Check sheet for the modelled part. Datum: model origin and axes. Units: mm. A direction names the side the tool comes from. Round coordinates to 2 decimals unless told otherwise and drop trailing zeros. Order: outer loops, then holes, each group sorted by start corner. A loop starts at its lowest first (then second) coordinate and runs counter-clockwise, first axis right, second up.
Q1. Cross-section at C-C on x = -22. Record the cut outline in (y, z), then the cut area to 3 significant figures.
Q2. Cross-section at B-B on z = 2.5. Record the cut outline in (x, y), then the cut area to 3 significant figures.
Q3. Cross-section at A-A on y = 20.5. Record the cut outline in (x, z), then the cut area to 3 significant figures.
Q4. Depth check by flat-ended pin: P1, Ø2.5, axis at x = 4, z = 2.5, coming from the +Y side. Enter the tip coordinate at first touch or a pass-through.
Q5. Mould release check, pull along X, two halves, no side actions. Record for faces 1 (the flat face through (0, 14, 0)), 2 (the flat face through (0, 15.955, 4)), 3 (the flat face through (-29.21, 20, 4)): +X half, -X half, draft (parallel to the pull), parting line (faces both ways), or undercut.
Q6. Cross-section at D-D on x = -10.5. Record the cut outline in (y, z), then the cut area to 3 significant figures.
Q7. Scan lines: probe 1 along X at (y, z) = (20.5, 5); probe 2 along Y at (x, z) = (-5, 5); probe 3 along Y at (x, z) = (22, 5). Record each from-to range of solid material in increasing order.
Q8. Set-up check for faces 4 (the flat face through (16.51, 33, 4)), 5 (the flat face through (29.21, 19, 4)): record each of +Z, -Z, +X, -X, +Y, -Y from which the full face is reachable in a straight line by a thin tool's end or side.
from build123d import *

# Parameters (mm, degrees)
F1_DEPTH = 7.62


with BuildPart() as f1:
    # F0 (on Top) → F1 (new body)
    with BuildSketch(Plane.XY):
        with BuildLine():
            Line((-29.210002, 48.974563), (-29.210002, 15.954563))
            Line((-29.210002, 15.954563), (-22.860002, 15.954563))
            Line((-22.860002, 15.954563), (-22.860002, 29.926767))
            ThreePointArc((-22.860002, 29.926767), (-25.397797, 32.464563), (-22.860002, 35.002358))
            Line((-22.860002, 35.002358), (-22.860002, 48.974563))
            Line((-22.860002, 48.974563), (-29.210002, 48.974563))
        make_face()
        Polygon((-22.860002, 15.954563), (-29.210002, 15.954563), (-29.210002, -9.445437), (29.209998, -9.445437), (29.209998, 15.954563), (22.859998, 15.954563), (16.509998, 15.954563), (-16.510002, 15.954563), align=None)
        with BuildLine():
            Line((-22.860002, 29.926767), (-22.860002, 15.954563))
            Line((-22.860002, 15.954563), (-16.510002, 15.954563))
            Line((-16.510002, 15.954563), (-16.510002, 48.974563))
            Line((-16.510002, 48.974563), (-22.860002, 48.974563))
            Line((-22.860002, 48.974563), (-22.860002, 35.002358))
            ThreePointArc((-22.860002, 35.002358), (-21.065509, 34.259055), (-20.322206, 32.464563))
            ThreePointArc((-20.322206, 32.464563), (-21.065509, 30.67007), (-22.860002, 29.926767))
        make_face()
        with BuildLine():
            Line((16.509998, 48.974563), (16.509998, 15.954563))
            Line((16.509998, 15.954563), (22.859998, 15.954563))
            Line((22.859998, 15.954563), (22.859998, 29.928652))
            ThreePointArc((22.859998, 29.928652), (20.324087, 32.464563), (22.859998, 35.000474))
            Line((22.859998, 35.000474), (22.859998, 48.974563))
            Line((22.859998, 48.974563), (16.509998, 48.974563))
        make_face()
        with BuildLine():
            Line((22.859998, 15.954563), (29.209998, 15.954563))
            Line((29.209998, 15.954563), (29.209998, 48.974563))
            Line((29.209998, 48.974563), (22.859998, 48.974563))
            Line((22.859998, 48.974563), (22.859998, 35.000474))
            ThreePointArc((22.859998, 35.000474), (24.653158, 34.257723), (25.395909, 32.464563))
            ThreePointArc((25.395909, 32.464563), (24.653158, 30.671403), (22.859998, 29.928652))
            Line((22.859998, 29.928652), (22.859998, 15.954563))
        make_face()
    extrude(amount=F1_DEPTH)


solid = f1.part
Results found:
1. outline: (-9.45, 0) - (30.08, 0) - (30.08, 7.62) - (-9.45, 7.62) - close; (34.85, 0) - (48.97, 0) - (48.97, 7.62) - (34.85, 7.62) - close
1. area: 409 mm2
2. outline: (-29.21, -9.45) - (29.21, -9.45) - (29.21, 48.97) - (16.51, 48.97) - (16.51, 15.95) - (-16.51, 15.95) - (-16.51, 48.97) - (-29.21, 48.97) - close; hole circle Ø5.08 at (-22.86, 32.46); hole circle Ø5.07 at (22.86, 32.46)
2. area: 2,280 mm2
3. outline: (-29.21, 0) - (-16.51, 0) - (-16.51, 7.62) - (-29.21, 7.62) - close; (16.51, 0) - (29.21, 0) - (29.21, 7.62) - (16.51, 7.62) - close
3. area: 194 mm2
4. P1: stops at y = 15.95
5. face 1: draft
5. face 2: undercut
5. face 3: -X half
6. outline: (-9.45, 0) - (15.95, 0) - (15.95, 7.62) - (-9.45, 7.62) - close
6. area: 194 mm2
7. probe 1: x = -29.21 to -16.51, 16.51 to 29.21
7. probe 2: y = -9.45 to 15.95
7. probe 3: y = -9.45 to 30.08, 34.85 to 48.97
8. face 4: +Z, -Z, +Y
8. face 5: +Z, -Z, +X, +Y, -Y
